Job drawing, mm, ordinate dimensions from the low corner. One solid piece. Give positions to 0.01 mm unless a question says otherwise; leave off trailing zeros. Order: outer loops, then holes, each group sorted by start corner. A loop starts at its lowest first (then second) coordinate and runs counter-clockwise, first axis right, second up. Notation, with made-up numbers: M -35.75,-24.5 L 19.25,-24.5 A31 ccw 19.25,9.5 Z; hole C -27.5,51 d1. An arc over 180 degrees is marked long. Put each result on its own line as item: value. Start each with the question number.
1) Drill centre lines: line 1 (Z direction, x = 18, y = 2); line 2 (X direction, y = 1.3, z = 8); line 3 (Z direction, x = 64, y = 2.55) (1 decimal). Where is each one in solid material? Low to high. Write a range as [from, to].
2) Cut at C-C (x = 105). Write the cut outline in (y, z), and give its area (3 significant figures).
3) Pin check, flat tips, straight feed: pin 1 (0.9 mm diameter, centred on y = 1.5, z = 10, fed in from +X); pin 2 (1.5 mm diameter, centred on y = 2, z = 62.5, fed in from -X); pin 3 (1 mm diameter, centred on x = 113.5, y = 1, fed in from +Z); pin 4 (2.5 mm diameter, centred on x = 125.5, z = 31.75, fed in from -Y). Stop position of each tip, or through.
4) Cut at B-B (y = 1.4). Give the number of separate pieces and of enclosed holes in the cut face, and give its area (3 significant figures).
5) Cut at D-D (z = 5). Write the cut outline in (x, y).
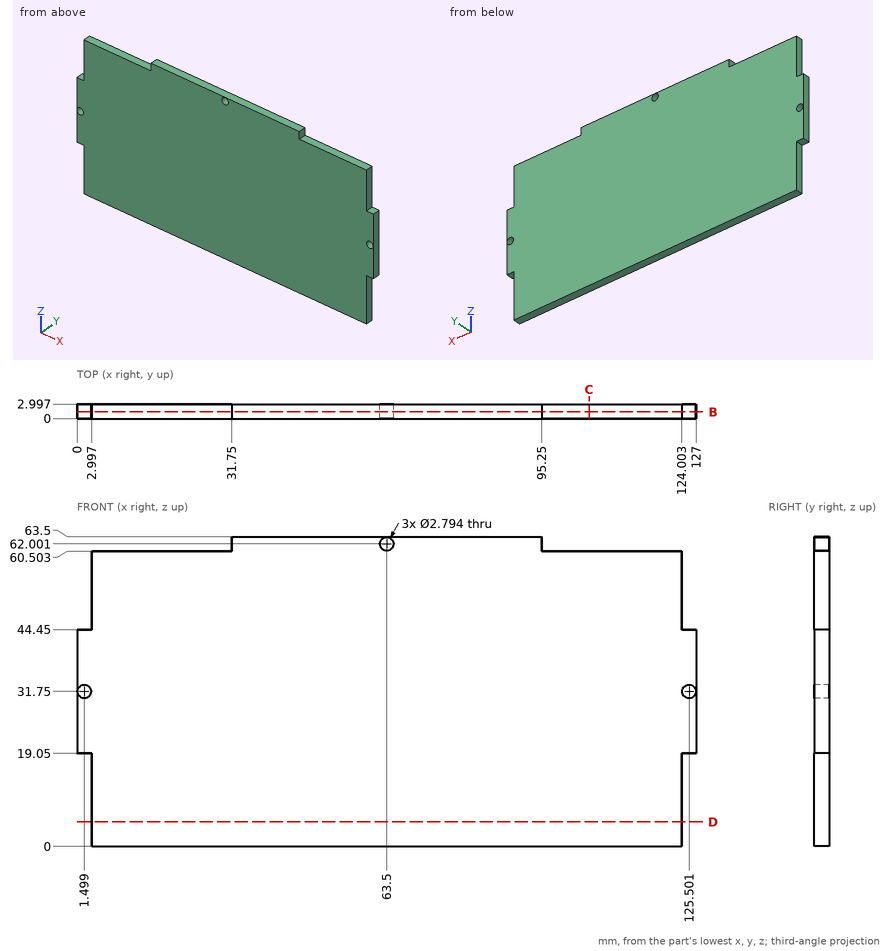
Solution:
1. line 1: [0, 60.5]
1. line 2: [3, 124]
1. line 3: [0, 60.7], [63.3, 63.5]
2. outline: M 0,0 L 3,0 L 3,60.5 L 0,60.5 Z
2. area: 181 mm²
3. pin 1: x = 124
3. pin 2: x = 31.75
3. pin 3: z = 60.5
3. pin 4: through
4. separate pieces: 1
4. enclosed holes: 3
4. area: 7,650 mm²
5. outline: M 3,0 L 124,0 L 124,3 L 3,3 Z
